```python
from build123d import *

# Parameters (mm, degrees)
F0_W     = 876.3
F0_H     = 38.1
F1_DEPTH = 9.652
F3_D     = 3.175
F3_DEPTH = 9.652
F4_R     = 12.7
F5_R     = 12.7
F6_W     = 876.3
F6_H     = 12.7
F7_DEPTH = 4.826


with BuildPart() as f1:
    # F0 (on Front) → F1 (new body)
    with BuildSketch(Plane.XZ):
        Rectangle(F0_W, F0_H)
    extrude(amount=F1_DEPTH)

    # F3
    with Locations(Plane(origin=(0, 0, 0), x_dir=(-1, 0, 0), z_dir=(0, 1, 0))):
        with Locations((-412.75, 6.35), (-234.95, 6.35), (0, 6.35), (234.95, 6.35), (412.75, 6.35)):
            Hole(F3_D / 2, depth=F3_DEPTH)

    # F4
    f4_edges = [f1.edges().sort_by_distance(p)[0] for p in [
        (438.15, -4.826, 19.05),
    ]]
    fillet(f4_edges, radius=F4_R)

    # F5
    f5_edges = [f1.edges().sort_by_distance(p)[0] for p in [
        (-438.15, -4.826, 19.05),
    ]]
    fillet(f5_edges, radius=F5_R)

    # F6 (on face) → F7 (cut)
    with BuildSketch(Plane.XZ.offset(9.652)):
        with Locations((0, -12.7)):
            Rectangle(F6_W, F6_H)
    extrude(amount=-F7_DEPTH, mode=Mode.SUBTRACT)


solid = f1.part
```
Check sheet for the modelled part. Datum: model origin and axes. Units: mm. Give positions to 0.01 mm unless a question says otherwise; leave off trailing zeros. Write each loop counter-clockwise with the first axis right and the second up, starting at its lowest first coordinate (ties: lowest second). Pieces come first, ordered by that corner, then holes. Notation, with made-up numbers: (10, -17) -> (34, -17) arc R14 ccw to (34, 6) -> close; hole circle Ø1 at (-21, -1). An arc over 180 degrees is marked (long way). Use CSV: the item, a comma, the result in double quotes. Start each with the question number.
Q1. Depth check by flat-ended pin: P1, Ø2, axis at x = 47.5, y = -7, coming from the -Z side; P2, Ø3, axis at y = -2, z = 13.5, coming from the +X side; P3, Ø6.5, axis at x = 192.5, z = -14, coming from the -Y side. Enter the tip coordinate at first touch or a pass-through.
Q2. Cross-section at A-A on x = 310. Enter the section's corners in (y, z).
Q3. Scan lines: line 1 along Z through (x, y) = (-412.75, -3.75); line 2 along Z through (x, y) = (0, -6.25); line 3 along Y through (x, z) = (-52.5, -8.5). Record each from-to range of solid material in increasing order.
Working result:
1,P1,"stops at z = -6.35"
1,P2,"stops at x = 436.82"
1,P3,"stops at y = -4.83"
2,outline,"(-9.65, -6.35) -> (-4.83, -6.35) -> (-4.83, -19.05) -> (0, -19.05) -> (0, 19.05) -> (-9.65, 19.05) -> close"
3,line 1,"z = -19.05 to 4.76, 7.94 to 19.05"
3,line 2,"z = -6.35 to 4.76, 7.94 to 19.05"
3,line 3,"y = -4.83 to 0"
